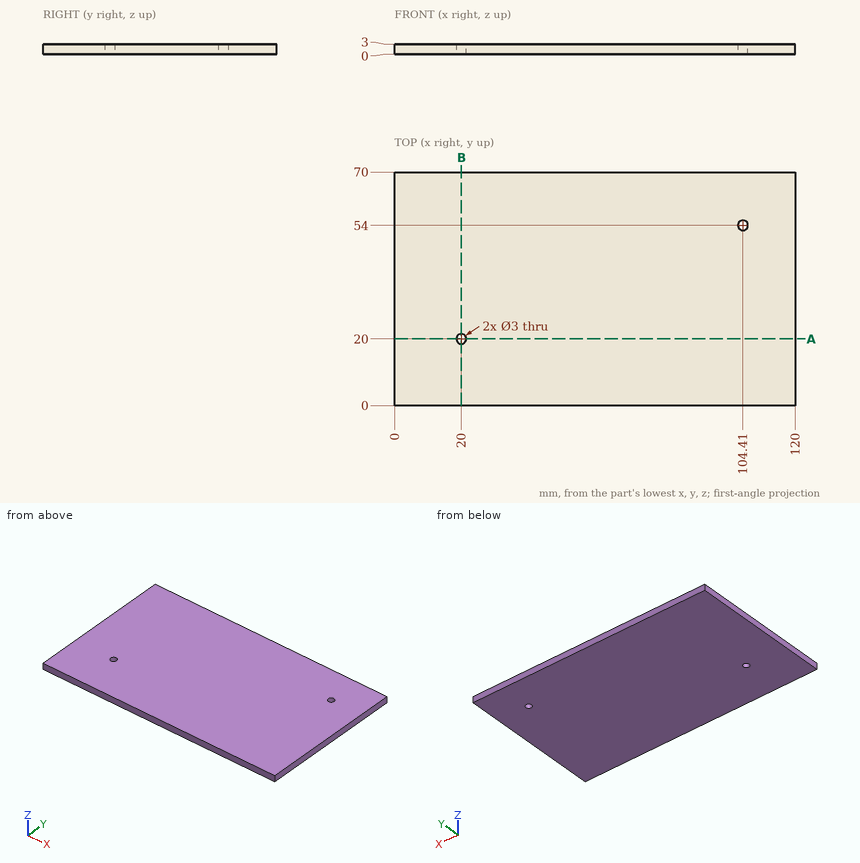
Geometry check sheet. Reference: drawing and pictorial views, mm from the part's lowest x, y, z. Coordinates: 2 decimals unless noted, no trailing zeros. Order: outer loops, then holes, each group sorted by start corner. A loop starts at its lowest first (then second) coordinate and runs counter-clockwise, first axis right, second up. Notation, with made-up numbers: (-10, 20) -> (-2, 20) arc R21 ccw to (-2, 29) -> close; hole circle Ø4 at (4.25, -39.5). An arc over 180 degrees is marked (long way). Write item = value, one per line. Start each with the question number.
1) Cross-section at B-B (x = 20). Enter the section's corners in (y, z), then the cut area to 3 significant figures.
2) Material ranges on L1, parallel to Y at x = 20, z = 1.05, recorded low to high.
3) Go/stop test with flat-tipped pins: P1, Ø2.5, axis at x = 20, y = 20, coming from the -Z side; P2, Ø1, axis at x = 46, z = 2, coming from the -Y side. Record where each tip stops, or that it passes through.
4) Cross-section at A-A (y = 20). Enter the section's corners in (x, z).
Ans:
q1.outline = (0, 0) -> (18.5, 0) -> (18.5, 3) -> (0, 3) -> close; (21.5, 0) -> (70, 0) -> (70, 3) -> (21.5, 3) -> close
q1.area = 201 mm²
q2.L1 = 0 to 18.5, 21.5 to 70
q3.P1 = through
q3.P2 = 0
q4.outline = (0, 0) -> (18.5, 0) -> (18.5, 3) -> (0, 3) -> close; (21.5, 0) -> (120, 0) -> (120, 3) -> (21.5, 3) -> close
